Here's how the part is built. I have some questions about the finished solid (model axes, mm). A direction names the side the tool comes from. Give positions to 0.01 mm unless a question says otherwise; leave off trailing zeros. Loops run counter-clockwise (first coordinate to the right, second up) from the corner with the lowest first, then second, coordinate; pieces in that order, holes last. Notation, with made-up numbers: (-21.5, -7.5) - (-17.5, -7.5) arc R12 cw to (-17.5, 7.5) - close; hole circle Ø3 at (-2.5, 8). An arc over 180 degrees is marked (long way). Use a Markdown table: item, result.
from build123d import *

# Parameters (mm, degrees)
F1_DEPTH = 50
F2_R     = 2.5
F3_DEPTH = 25
F4_R     = 2


with BuildPart() as f1:
    # F0 (on Top) → F1 (new body)
    with BuildSketch(Plane.XY):
        Polygon((-41, -15), (34, -15), (34, -35), (41, -35), (41, -15), (41, 0), (-36, 0), (-36, 15), (-41, 15), align=None)
    extrude(amount=F1_DEPTH)

    # F2 (on face) → F3 (cut)
    with BuildSketch(Plane(origin=(34, 0, 0), x_dir=(0, -1, 0), z_dir=(-1, 0, 0))):
        with Locations((25, 12)):
            Circle(F2_R)
        with Locations((25, 38)):
            Circle(F2_R)
    extrude(amount=-F3_DEPTH, mode=Mode.SUBTRACT)

    # F4
    f4_edges = [f1.edges().sort_by_distance(p)[0] for p in [
        (-3.5, -15, 50),
        (34, -25, 50),
        (37.5, -35, 50),
        (41, -17.5, 50),
        (2.5, 0, 50),
        (-36, 7.5, 50),
        (-38.5, 15, 50),
        (-41, 0, 50),
        (-3.5, -15, 0),
        (34, -25, 0),
        (37.5, -35, 0),
        (41, -17.5, 0),
        (2.5, 0, 0),
        (-36, 7.5, 0),
        (-38.5, 15, 0),
        (-41, 0, 0),
        (34, -35, 25),
        (-41, -15, 25),
        (-41, 15, 25),
        (-36, 15, 25),
        (41, 0, 25),
        (-36, 0, 25),
        (41, -35, 25),
    ]]
    fillet(f4_edges, radius=F4_R)


solid = f1.part
(1) Suppose I cut it at D-D on z = 34. Write out the boundary of the cut face in (x, y).
A:
| item | result |
|---|---|
| outline | (-41, -13) arc R2 ccw to (-39, -15) - (34, -15) - (34, -33) arc R2 ccw to (36, -35) - (39, -35) arc R2 ccw to (41, -33) - (41, -2) arc R2 ccw to (39, 0) - (-34, 0) arc R2 cw to (-36, 2) - (-36, 13) arc R2 ccw to (-38, 15) - (-39, 15) arc R2 ccw to (-41, 13) - close |
(2) Suppose I cut it at B-B on z = 12. Write out the boundary of the cut face in (x, y).
A:
| item | result |
|---|---|
| outline | (-41, -13) arc R2 ccw to (-39, -15) - (34, -15) - (34, -22.5) - (41, -22.5) - (41, -2) arc R2 ccw to (39, 0) - (-34, 0) arc R2 cw to (-36, 2) - (-36, 13) arc R2 ccw to (-38, 15) - (-39, 15) arc R2 ccw to (-41, 13) - close; (34, -33) arc R2 ccw to (36, -35) - (39, -35) arc R2 ccw to (41, -33) - (41, -27.5) - (34, -27.5) - close |
(3) On a 3-axis mill with a long thin cutter (end or side, diameter ignored), from which of +Z, -Z, +X, -X, +Y, -Y can I reach the whole of each face in a straight line? I mean faces 1 (the face through (1.99, -0.6, 49.43)), 2 (the face through (1.99, -0.6, 0.57)), 3 (the face through (-0.97, -14.43, 49.4)), 4 (the face through (-3, -15, 25)), 5 (the face through (3, 0, 25)). Say none if no direction works.
A:
| item | result |
|---|---|
| face 1 | +Z, +X, +Y |
| face 2 | -Z, +X, +Y |
| face 3 | +Z, -X, -Y |
| face 4 | +Z, -Z, -X, -Y |
| face 5 | +Z, -Z, +X, +Y |
(4) Suppose I cut it at C-C on y = -17. Write out the boundary of the cut face in (x, z).
A:
| item | result |
|---|---|
| outline | (34, 2) arc R2 ccw to (36, 0) - (39, 0) arc R2 ccw to (41, 2) - (41, 48) arc R2 ccw to (39, 50) - (36, 50) arc R2 ccw to (34, 48) - close |
(5) We'd pull the mould along Y, two halves only. Please class faces 6 (the face through (-36.6, 14.43, 25.32)), 7 (the face through (37.52, -34.4, 49.43)), 8 (the face through (34.57, -23.14, 49.4)), 9 (the face through (37.45, -24.46, 9.56)): pulls with the +Y half, pulls with the -Y half, needs draft (parallel to the pull), parting line crosses it, or undercut.
A:
| item | result |
|---|---|
| face 6 | pulls with the +Y half |
| face 7 | pulls with the -Y half |
| face 8 | needs draft |
| face 9 | undercut |
(6) Suppose I cut it at A-A on y = -25. Write out the boundary of the cut face in (x, z).
A:
| item | result |
|---|---|
| outline | (34, 2) arc R2 ccw to (36, 0) - (39, 0) arc R2 ccw to (41, 2) - (41, 9.5) - (34, 9.5) - close; (34, 14.5) - (41, 14.5) - (41, 35.5) - (34, 35.5) - close; (34, 40.5) - (41, 40.5) - (41, 48) arc R2 ccw to (39, 50) - (36, 50) arc R2 ccw to (34, 48) - close |
(7) If I drill on line 1 (Z direction, x = 36.5, y = -25); line 2 (Z direction, x = 39.75, y = -25); line 3 (X direction, y = -28.5, z = 24), over which ranges is the centre line in solid material (lowest first)?
A:
| item | result |
|---|---|
| line 1 | 0 to 9.5, 14.5 to 35.5, 40.5 to 50 |
| line 2 | 0.15 to 9.5, 14.5 to 35.5, 40.5 to 49.85 |
| line 3 | 34 to 41 |
(8) Will these pins go through, and if not, where does the flat tip stop? pin 1 (3 mm diameter, centred on x = 7.5, z = 14.5, fed in from -Y); pin 2 (1 mm diameter, centred on x = -6, y = 1, fed in from -Z); pin 3 (9 mm diameter, centred on y = 9, z = 25.5, fed in from +X); pin 4 (1 mm diameter, centred on x = -3, z = 21.5, fed in from +Y).
A:
| item | result |
|---|---|
| pin 1 | y = -15 |
| pin 2 | through |
| pin 3 | x = -36 |
| pin 4 | y = 0 |
